from build123d import *

# Parameters (mm, degrees)
SKETCH1_R           = 23.5
SKETCH1_R_2         = 22.5
EXTRUDE_THIN1_DEPTH = 12
BOSS_EXTRUDE2_DEPTH = 12
CIRPATTERN4_COUNT   = 30


with BuildPart() as part:
    # Sketch1 → Extrude-Thin1 (new body)
    with BuildSketch(Plane(origin=(0, 0, 0), x_dir=(0, 0, -1), z_dir=(1, 0, 0))):
        Circle(SKETCH1_R)
        Circle(SKETCH1_R_2, mode=Mode.SUBTRACT)
    extrude(amount=EXTRUDE_THIN1_DEPTH)

    # Sketch3 → Boss-Extrude2 (add)
    with BuildSketch(Plane.ZY):
        Polygon((-1, 24.452078799), (1, 24.452078799), (1.5, 23.452078799), (-1.5, 23.452078799), align=None)
    boss_extrude2 = extrude(amount=-BOSS_EXTRUDE2_DEPTH)

    # CirPattern4: Boss-Extrude2 ×30 about axis
    cirpattern4_axis = Axis((0, 0, 0), (1, 0, 0))
    for i in range(1, CIRPATTERN4_COUNT):
        add(boss_extrude2.rotate(cirpattern4_axis, i * 360 / CIRPATTERN4_COUNT))


solid = part.part
Build history of the part. All positions in model axes, mm. A direction names the side the tool comes from. Give positions to 0.01 mm unless a question says otherwise; leave off trailing zeros. Loops run counter-clockwise (first coordinate to the right, second up) from the corner with the lowest first, then second, coordinate; pieces in that order, holes last. Notation, with made-up numbers: (70, 71) - (103, 71) arc R27 ccw to (103, 102) - close; hole circle Ø11 at (-36.5, 4.25). An arc over 180 degrees is marked (long way). Write item = value, one per line. Start each with the question number.
1) Drop flat-ended pins along their axis: pin 1 Ø2 at (x, y) = (8.5, 12) entering from +Z; pin 2 Ø5 at (x, y) = (9.5, -9) entering from -Z; pin 3 Ø1.5 at (x, z) = (3.5, -13) entering from +Y. Give the stop position or say it passes through.
2) Tool access for faces 1 (the cylindrical face through (5.92, 23.37, -2.47)), 2 (the flat face through (5.916, -16.958, 16.971)), 3 (the cylindrical face through (5.92, -9.55, 21.47)): list every direction of +Z, -Z, +X, -X, +Y, -Y with a clear straight run to the whole face (end or side of a thin tool).
3) Probe probe 1 along Y at (x, z) = (7.75, 0); probe 2 along Y at (x, z) = (7, -6); probe 3 along Z at (x, y) = (1, -16.5). List the from-to ranges inside material, lowest first. Write a range as from..to.
4) Pull direction Y, two halves, no side cores. Call faces 4 (the flat face through (5.92, -8.59, -22.39)), 5 (the cylindrical face through (5.916, 20.358, 11.738)), 6 (the cylindrical face through (5.916, -4.899, -22.984)): +Y half, -Y half, draft (parallel to the pull), parting line (faces both ways), or undercut.
5) Band-saw the part on A-A on y = 0. Give the cut face in (x, z).
6) Band-saw the part on B-B on z = 0. Give the cut face in (x, y).
Final values:
q1.pin_1 = 21.68
q1.pin_2 = -23.56
q1.pin_3 = 20.37
q2.face_1 = +X, -X, +Y
q2.face_2 = +X, -X, -Y
q2.face_3 = +Z, +X, -X
q3.probe_1 = -24.45..-22.5, 22.5..24.45
q3.probe_2 = -23.72..-21.69, 21.69..23.72
q3.probe_3 = -18.05..-15.3, 15.3..18.05
q4.face_4 = -Y half
q4.face_5 = +Y half
q4.face_6 = undercut
q5.outline = (0, -23.5) - (12, -23.5) - (12, -22.5) - (0, -22.5) - close; (0, 22.5) - (12, 22.5) - (12, 23.5) - (0, 23.5) - close
q6.outline = (0, -24.45) - (12, -24.45) - (12, -22.5) - (0, -22.5) - close; (0, 22.5) - (12, 22.5) - (12, 24.45) - (0, 24.45) - close
